Work out the finished part from the listing and answer in its coordinate system (mm). Face numbers are marked on the shaded views. A direction names the side the tool comes from. Give positions to 0.01 mm unless a question says otherwise; leave off trailing zeros. Loops run counter-clockwise (first coordinate to the right, second up) from the corner with the lowest first, then second, coordinate; pieces in that order, holes last. Notation, with made-up numbers: (-8, 5.25) -> (-4, 5.25) arc R21 cw to (-4, 31.25) -> close; hole circle Ø9 at (-20, 81.25). An arc over 180 degrees is marked (long way). Answer as CSV lines item,"result". Start each with the question number.
1. Find section C-C, the plane z = -308. Give the vertices of the cut face in (x, y).
2. Find section A-A, the plane x = 40.75. Give the vertices of the cut face in (y, z).
3. Flat-ended cylindrical pins translate along their axes: pin 1 Ø6 at (y, z) = (-79.5, -307) entering from +X; pin 2 Ø5 at (x, z) = (46.03, -313.01) entering from +Y; pin 3 Ø4 at (x, z) = (46.5, -253.5) entering from -Y. Find the tip coordinate at first contact, or state that the pin passes through.
4. A tool of negligible diameter and unlimited length cuts with its end or side. For the marked faces 1, 2, 3, 4 and 5, from which of +Z, -Z, +X, -X, +Y, -Y can it reach the whole face along a straight path? Write none if from no direction.
5. Find section B-B, the plane y = -99.5. Give the vertices of the cut face in (x, z) (3 decimals).
6. Find section D-D, the plane x = 48.5. Give the vertices of the cut face in (y, z), and give its area (3 significant figures).
7. Find the intervals of material crossed by line 1 along Y through (x, z) = (33.75, -295); line 2 along Z through (x, y) = (41.5, -99.5); line 3 along X through (y, z) = (-68.5, -301), in increasing order.
8. Determine the mould class of the marked faces 6, 7 and 8 for opening direction X: +X half, -X half, draft (parallel to the pull), parting line (faces both ways), or undercut.
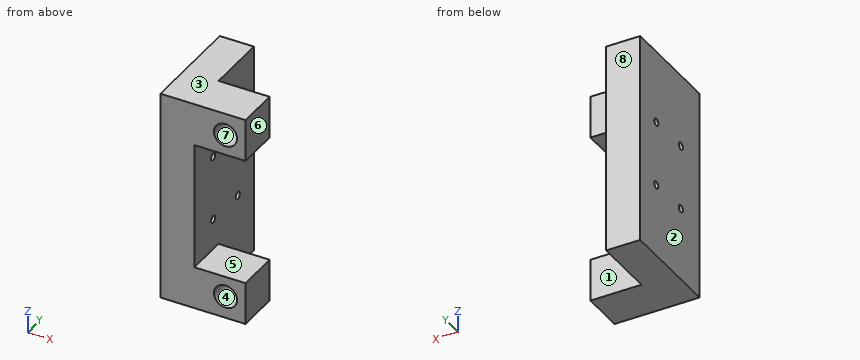
from build123d import *

# Parameters (mm, degrees)
SKETCH1_W           = 74.870479659
SKETCH1_H           = 36.98000569
BOSS_EXTRUDE1_DEPTH = 12
SKETCH4_W           = 15
SKETCH4_H           = 15
BOSS_EXTRUDE3_DEPTH = 18
SKETCH5_R           = 4.075
CUT_EXTRUDE1_DEPTH  = 12
SKETCH3_R           = 1.27
CUT_EXTRUDE3_DEPTH  = 13


with BuildPart() as part:
    # Sketch1 → Boss-Extrude1 (new body)
    with BuildSketch(Plane.ZY.offset(-35.076450848)):
        with Locations((-283.368991002, -85.966002845)):
            Rectangle(SKETCH1_W, SKETCH1_H)
    extrude(amount=BOSS_EXTRUDE1_DEPTH)

    # Sketch4 → Boss-Extrude3 (add)
    with BuildSketch(Plane(origin=(35.076450848, 0, 0), x_dir=(0, 0, -1), z_dir=(1, 0, 0))):
        with Locations((253.433751172, -96.95600569)):
            Rectangle(SKETCH4_W, SKETCH4_H)
        with Locations((313.304230831, -96.95600569)):
            Rectangle(SKETCH4_W, SKETCH4_H)
    extrude(amount=BOSS_EXTRUDE3_DEPTH)

    # Sketch5 → Cut-Extrude1 (cut)
    with BuildSketch(Plane.XZ.offset(104.45600569)):
        with Locations((46.026450848, -253.725)):
            Circle(SKETCH5_R)
        with Locations((46.026450848, -313.012982003)):
            Circle(SKETCH5_R)
    extrude(amount=-CUT_EXTRUDE1_DEPTH, mode=Mode.SUBTRACT)

    # Sketch3 → Cut-Extrude3 (cut, through all)
    with BuildSketch(Plane(origin=(35.076450848, 0, 0), x_dir=(0, 0, -1), z_dir=(1, 0, 0))):
        with Locations((271.868893694, -77.476)):
            Circle(SKETCH3_R)
        with Locations((271.868893694, -92.776)):
            Circle(SKETCH3_R)
        with Locations((294.868893694, -77.476)):
            Circle(SKETCH3_R)
        with Locations((294.868893694, -92.776)):
            Circle(SKETCH3_R)
    extrude(amount=-CUT_EXTRUDE3_DEPTH, mode=Mode.SUBTRACT)


solid = part.part
Resolved:
1,outline,"(23.08, -104.46) -> (53.08, -104.46) -> (53.08, -89.46) -> (35.08, -89.46) -> (35.08, -67.48) -> (23.08, -67.48) -> close"
2,outline,"(-104.46, -320.8) -> (-89.46, -320.8) -> (-89.46, -305.8) -> (-104.46, -305.8) -> close; (-104.46, -260.93) -> (-89.46, -260.93) -> (-89.46, -245.93) -> (-104.46, -245.93) -> close"
3,pin 1,"stops at x = 35.08"
3,pin 2,"stops at y = -89.46"
3,pin 3,"stops at y = -92.46"
4,face 1,"+Z, -Z, +X, +Y"
4,face 2,"+Z, -Z, -X, +Y, -Y"
4,face 3,"+Z, +X, -X, +Y, -Y"
4,face 4,"-Y"
4,face 5,"+X, +Y, -Y"
5,outline,"(23.076, -320.804) -> (53.076, -320.804) -> (53.076, -305.804) -> (35.076, -305.804) -> (35.076, -260.934) -> (53.076, -260.934) -> (53.076, -245.934) -> (23.076, -245.934) -> close; hole circle Ø8.15 at (46.026, -313.013); hole circle Ø8.15 at (46.026, -253.725)"
6,outline,"(-104.46, -320.8) -> (-89.46, -320.8) -> (-89.46, -305.8) -> (-104.46, -305.8) -> (-104.46, -309.77) -> (-92.46, -309.77) -> (-92.46, -316.25) -> (-104.46, -316.25) -> close; (-104.46, -260.93) -> (-89.46, -260.93) -> (-89.46, -245.93) -> (-104.46, -245.93) -> (-104.46, -250.49) -> (-92.46, -250.49) -> (-92.46, -256.96) -> (-104.46, -256.96) -> close"
6,area,"295 mm^2"
7,line 1,"y = -104.46 to -94.04, -91.51 to -78.74, -76.21 to -67.48"
7,line 2,"z = -320.8 to -305.8, -260.93 to -245.93"
7,line 3,"x = 23.08 to 35.08"
8,face 6,"+X half"
8,face 7,"undercut"
8,face 8,"draft"
